Work out the finished part from the listing and answer in its coordinate system (mm). Face numbers are marked on the shaded views. A direction names the side the tool comes from. Coordinates: 2 decimals unless noted, no trailing zeros. Loops run counter-clockwise (first coordinate to the right, second up) from the corner with the lowest first, then second, coordinate; pieces in that order, holes last. Notation, with made-up numbers: (45, 78) -> (69, 78) arc R13 cw to (69, 100) -> close; hole circle Ø3 at (10, 32). An arc over 180 degrees is marked (long way). Use a Markdown table: item, result.
from build123d import *

# Parameters (mm, degrees)
F0_R     = 6.35
F1_DEPTH = 25.4
F2_R     = 5.08
F3_R     = 5.08


with BuildPart() as f1:
    # F0 (on Right) → F1 (new body)
    with BuildSketch(Plane.YZ):
        with BuildLine():
            Line((44.45, 0), (19.05, 0))
            ThreePointArc((19.05, 0), (0, 19.05), (-19.05, 0))
            Line((-19.05, 0), (-44.45, 0))
            Line((-44.45, 0), (-44.45, -19.05))
            Line((-44.45, -19.05), (44.45, -19.05))
            Line((44.45, -19.05), (44.45, 0))
        make_face()
        Circle(F0_R, mode=Mode.SUBTRACT)
    extrude(amount=F1_DEPTH)

    # F2
    f2_edges = [f1.edges().sort_by_distance(p)[0] for p in [
        (12.7, 44.45, 0),
    ]]
    fillet(f2_edges, radius=F2_R)

    # F3
    f3_edges = [f1.edges().sort_by_distance(p)[0] for p in [
        (12.7, -44.45, 0),
    ]]
    fillet(f3_edges, radius=F3_R)


solid = f1.part
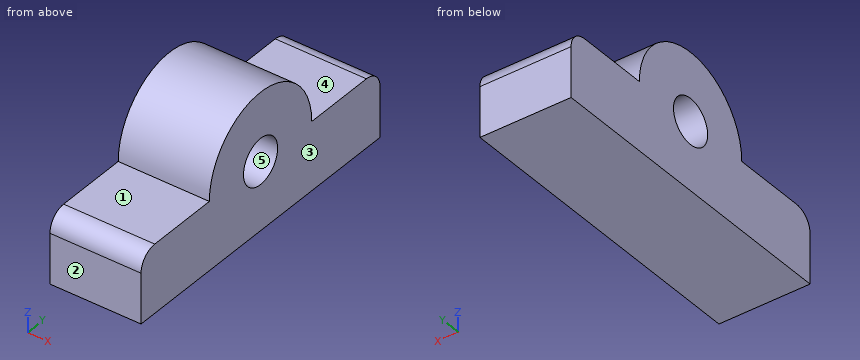
Q1. Section B-B on y = 0 is taken. Determine the outline of the cut face in (x, z), and give its area (3 significant figures).
Solved:
| item | result |
|---|---|
| outline | (0, -19.05) -> (25.4, -19.05) -> (25.4, -6.35) -> (0, -6.35) -> close; (0, 6.35) -> (25.4, 6.35) -> (25.4, 19.05) -> (0, 19.05) -> close |
| area | 645 mm² |
Q2. Determine the mould class of the marked faces 3, 4 and 5 for opening direction Z: pulls with the +Z half, pulls with the -Z half, needs draft (parallel to the pull), parting line crosses it, or undercut.
Solved:
| item | result |
|---|---|
| face 3 | needs draft |
| face 4 | pulls with the +Z half |
| face 5 | undercut |
Q3. Section A-A on x = 9.25 is taken. Determine the outline of the cut face in (y, z).
Solved:
| item | result |
|---|---|
| outline | (-44.45, -19.05) -> (44.45, -19.05) -> (44.45, -5.08) arc R5.08 ccw to (39.37, 0) -> (19.05, 0) arc R19.05 ccw to (-19.05, 0) -> (-39.37, 0) arc R5.08 ccw to (-44.45, -5.08) -> close; hole circle Ø12.7 at (0, 0) |
Q4. Section C-C on z = 14.5 is taken. Determine the outline of the cut face in (x, y).
Solved:
| item | result |
|---|---|
| outline | (0, -12.36) -> (25.4, -12.36) -> (25.4, 12.36) -> (0, 12.36) -> close |
Q5. Section D-D on y = 28.5 is taken. Determine the outline of the cut face in (x, z), and give its area (3 significant figures).
Solved:
| item | result |
|---|---|
| outline | (0, -19.05) -> (25.4, -19.05) -> (25.4, 0) -> (0, 0) -> close |
| area | 484 mm² |
Q6. Given pin 1 Ø4 at (x, y) = (10, 28.5) entering from +Z; pin 2 Ø3 at (y, z) = (-5, -10) entering from -X; pin 3 Ø1 at (x, z) = (5, 11) entering from -Y; pin 4 Ø12 at (x, y) = (14.5, 18) entering from +Z, each flat-ended and moving along its own axis, determine where each tip first touches the part or whether it passes through.
Solved:
| item | result |
|---|---|
| pin 1 | z = 0 |
| pin 2 | x = 0 |
| pin 3 | y = -15.9 |
| pin 4 | z = 14.8 |
Q7. Consider line 1 (Z direction, x = 18, y = 0); line 2 (Y direction, x = 3, z = -5.5); line 3 (Y direction, x = 7, z = -2.5). Determine where each line is inside the solid, lowest interval first. Write a range as [from, to].
Solved:
| item | result |
|---|---|
| line 1 | [-19.05, -6.35], [6.35, 19.05] |
| line 2 | [-44.45, -3.17], [3.17, 44.45] |
| line 3 | [-43.75, -5.84], [5.84, 43.75] |
Q8. For the marked faces 1 and 2, determine the directions among +Z, -Z, +X, -X, +Y, -Y from which every point of the face is accessible in a straight line to the end or side of a thin tool.
Solved:
| item | result |
|---|---|
| face 1 | +Z, +X, -X, -Y |
| face 2 | +Z, -Z, +X, -X, -Y |
